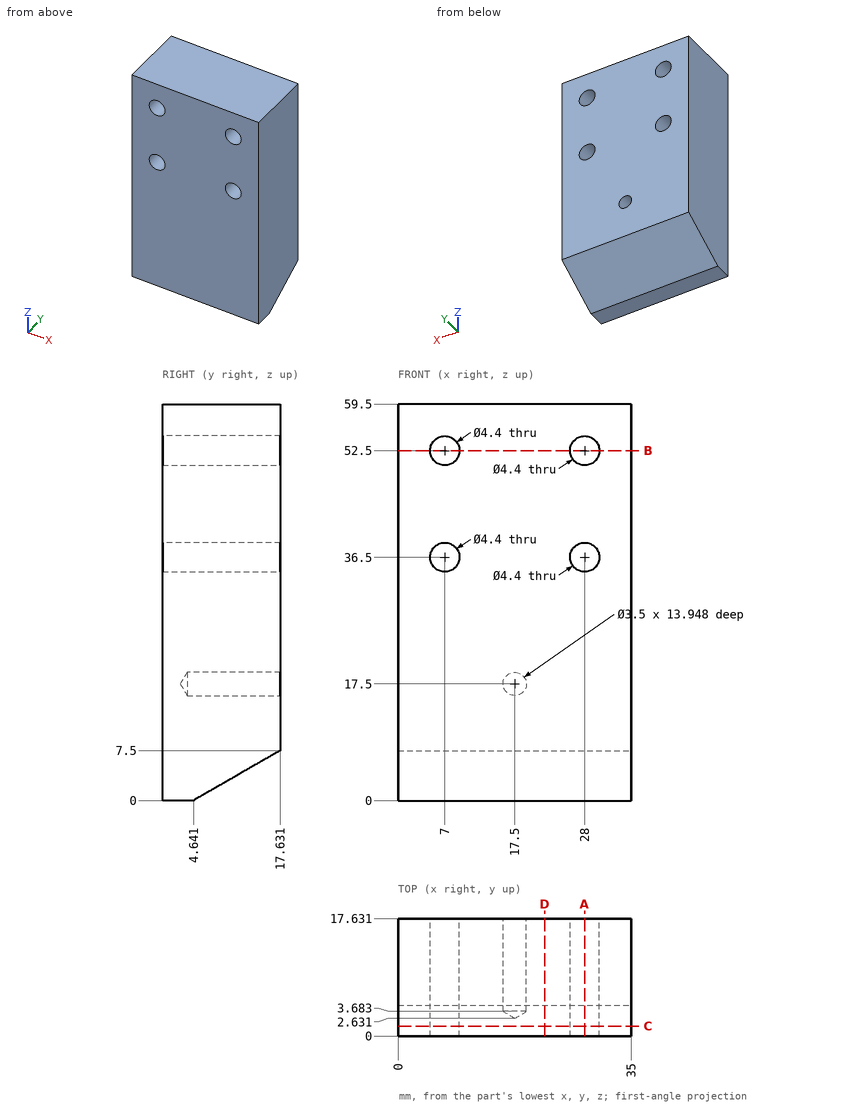
Study the drawing (mm; zero at the part's minimum x, y, z) and answer. Round coordinates to 2 decimals unless told otherwise and drop trailing zeros. Write each loop counter-clockwise with the first axis right and the second up, starting at its lowest first coordinate (ties: lowest second). Pieces come first, ordered by that corner, then holes. Notation, with made-up numbers: (2, 3.5) -> (14, 3.5) arc R15 ccw to (14, 9.5) -> close; hole circle Ø3 at (76.5, -17). An arc over 180 degrees is marked (long way). Write item = value, one per line.
1) Section C-C on y = 1.5 is taken. Write down the section's boundary in (x, z), plus the area to 3 significant figures.
Check values:
outline = (0, 0) -> (35, 0) -> (35, 59.5) -> (0, 59.5) -> close; hole circle Ø4.4 at (7, 36.5); hole circle Ø4.4 at (7, 52.5); hole circle Ø4.4 at (28, 36.5); hole circle Ø4.4 at (28, 52.5)
area = 2,020 mm²
2) Straight lines are drawn through the part: line 1 along X through (y, z) = (5.5, 36.5); line 2 along Z through (x, y) = (9, 10.5) (1 decimal); line 3 along X through (y, z) = (7.25, 17.5). For each, find the intervals that lie inside material, in ascending order. Write a range as [from, to].
Check values:
line_1 = [0, 4.8], [9.2, 25.8], [30.2, 35]
line_2 = [3.4, 35.6], [37.4, 51.6], [53.4, 59.5]
line_3 = [0, 15.75], [19.25, 35]
3) Given pin 1 (4 mm diameter, centred on x = 27.5, y = 13, fed in from -Z); pin 2 (3 mm diameter, centred on x = 17.5, z = 17.5, fed in from -Y); pin 3 (10 mm diameter, centred on x = 19.5, y = 10, fed in from -Z); pin 4 (3.5 mm diameter, centred on x = 28, z = 52.5, fed in from +Y), each flat-ended and moving along its own axis, determine where each tip first touches the part or whether it passes through.
Check values:
pin_1 = 3.67
pin_2 = 0
pin_3 = 0.21
pin_4 = through
4) Section D-D on x = 22 is taken. Write down the section's boundary in (y, z), plus the area to 3 significant figures.
Check values:
outline = (0, 0) -> (4.64, 0) -> (17.63, 7.5) -> (17.63, 59.5) -> (0, 59.5) -> close
area = 1,000 mm²
5) Section B-B on z = 52.5 is taken. Write down the section's boundary in (x, y).
Check values:
outline = (0, 0) -> (4.8, 0) -> (4.8, 17.63) -> (0, 17.63) -> close; (9.2, 0) -> (25.8, 0) -> (25.8, 17.63) -> (9.2, 17.63) -> close; (30.2, 0) -> (35, 0) -> (35, 17.63) -> (30.2, 17.63) -> close
6) Section A-A on x = 28 is taken. Write down the section's boundary in (y, z).
Check values:
outline = (0, 0) -> (4.64, 0) -> (17.63, 7.5) -> (17.63, 34.3) -> (0, 34.3) -> close; (0, 38.7) -> (17.63, 38.7) -> (17.63, 50.3) -> (0, 50.3) -> close; (0, 54.7) -> (17.63, 54.7) -> (17.63, 59.5) -> (0, 59.5) -> close
